```python
from build123d import *

# Parameters (mm, degrees)
BOSS_EXTRUDE1_DEPTH   = 6.35
F_6_CLEARANCE_HOLE1_D = 3.6576


with BuildPart() as part:
    # Sketch1 → Boss-Extrude1 (new body)
    with BuildSketch(Plane.XY):
        Polygon((0, 0), (0, 4.5), (5.5, 4.5), (5.5, 13), (28.5, 13), (28.5, 4.5), (34, 4.5), (34, 0), (23.25, 0), (23.25, 3.75), (10.75, 3.75), (10.75, 0), align=None)
    extrude(amount=BOSS_EXTRUDE1_DEPTH)

    # #6 Clearance Hole1 (through all)
    with Locations(Plane(origin=(26.25, 13, 3.175), x_dir=(0, 0, 1), z_dir=(0, 1, 0))):
        with Locations((0, 0), (0, -18.5)):
            Hole(F_6_CLEARANCE_HOLE1_D / 2)


solid = part.part
```
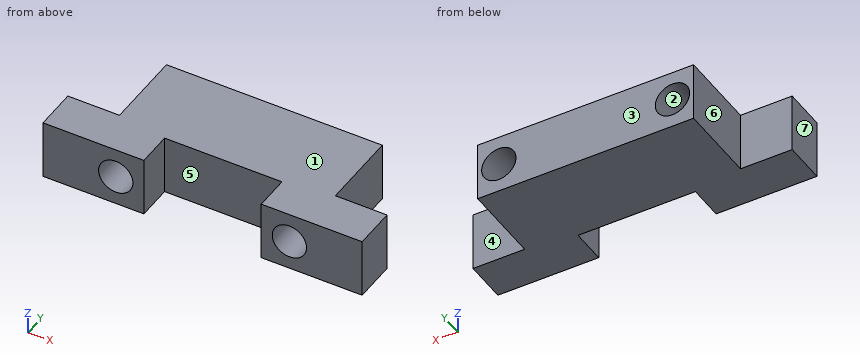
Input: part model. Units: mm. Frame: model coordinates. Face numbers are marked on the shaded views. A direction names the side the tool comes from. Coordinates: 2 decimals unless noted, no trailing zeros. Loops run counter-clockwise (first coordinate to the right, second up) from the corner with the lowest first, then second, coordinate; pieces in that order, holes last. Notation, with made-up numbers: M 22.5,41.5 L 40.5,41.5 A22 cw 40.5,50.5 Z; hole C 69.25,51 d9. An arc over 180 degrees is marked long. Use a Markdown table: item, result. Add a question column.
1) Set-up query: the marked faces 4, 5, 6 and 7. Return all of +Z, -Z, +X, -X, +Y, -Y with unobstructed straight access to the full face (end or side cutting, diameter ignored); none if empty.
2) Line query: L1, parallel to X at y = 8, z = 3.25; L2, parallel to X at y = 2.75, z = 4.75; L3, parallel to X at y = 11.25, z = 4.75. Output: solid intervals per line, ascending. Write a range as from..to.
3) Section B-B, the plane x = 26.25. Return the cut outline in (y, z), plus the area to 3 significant figures.
4) Draft query along Z for the marked faces 1, 2 and 3. Return one class per face: +Z half, -Z half, draft (parallel to the pull), parting line (faces both ways), or undercut.
5) Section D-D, the plane y = 7.5. Return the cut outline in (x, z) (3 decimals).
6) Section C-C, the plane z = 1. Return the cut outline in (x, y), plus the area to 3 significant figures.
7) Pin query (flat end, axial travel): P1, Ø1.9, axis at x = 17.5, z = 4.5, coming from the -Y side. Return the tip coordinate at first contact, or that it passes through.
8) Section A-A, the plane y = 1.25. Return the cut outline in (x, z) (3 decimals).
Answer below:
| question | item | result |
|---|---|---|
| 1 | face 4 | +Z, -Z, +X, +Y |
| 1 | face 5 | +Z, -Z, -Y |
| 1 | face 6 | +Z, -Z, -X, +Y |
| 1 | face 7 | +Z, -Z, -X, +Y, -Y |
| 2 | L1 | 5.5..5.92, 9.58..24.42, 28.08..28.5 |
| 2 | L2 | 0..6.82, 8.68..10.75, 23.25..25.32, 27.18..34 |
| 2 | L3 | 5.5..6.82, 8.68..25.32, 27.18..28.5 |
| 3 | outline | M 0,0 L 13,0 L 13,1.35 L 0,1.35 Z; M 0,5 L 13,5 L 13,6.35 L 0,6.35 Z |
| 3 | area | 35.0 mm2 |
| 4 | face 1 | +Z half |
| 4 | face 2 | undercut |
| 4 | face 3 | draft |
| 5 | outline | M 5.5,0 L 28.5,0 L 28.5,6.35 L 5.5,6.35 Z; hole C 7.75,3.175 d3.658; hole C 26.25,3.175 d3.658 |
| 6 | outline | M 0,0 L 10.75,0 L 10.75,3.75 L 23.25,3.75 L 23.25,0 L 34,0 L 34,4.5 L 28.5,4.5 L 28.5,13 L 5.5,13 L 5.5,4.5 L 0,4.5 Z |
| 6 | area | 302 mm2 |
| 7 | P1 | y = 3.75 |
| 8 | outline | M 0,0 L 10.75,0 L 10.75,6.35 L 0,6.35 Z; M 23.25,0 L 34,0 L 34,6.35 L 23.25,6.35 Z; hole C 7.75,3.175 d3.658; hole C 26.25,3.175 d3.658 |
